Verification items for the finished model (mm, model axes). A direction names the side the tool comes from. Round coordinates to 2 decimals unless told otherwise and drop trailing zeros. Write each loop counter-clockwise with the first axis right and the second up, starting at its lowest first coordinate (ties: lowest second). Pieces come first, ordered by that corner, then holes. Notation, with made-up numbers: M 71.25,-5 L 97.25,-5 A27 ccw 97.25,19 Z; hole C 33.25,84.25 d1. An arc over 180 degrees is marked long. Answer in a Markdown table with one row per item. Add a question column.
1. Sectioned sample at A-A on y = 63.5. Record the cut outline in (x, z).
2. Go/stop test with flat-tipped pins: pin 1 Ø3.5 at (x, y) = (-41, 63.5) entering from -Z; pin 2 Ø1.6 at (y, z) = (67.5, -8) entering from -X; pin 3 Ø6 at (x, z) = (-35, -6) entering from -Y. Record where each tip stops, or that it passes through.
3. Sectioned sample at C-C on z = -7.25. Record the cut outline in (x, y).
4. Sectioned sample at D-D on x = -54. Record the cut outline in (y, z), plus the area to 3 significant figures.
5. Sectioned sample at B-B on x = -27. Record the cut outline in (y, z).
6. Draft check along Y on faces 1 (the cylindrical face through (-48.162, 64.215, 3.944)), 2 (the cylindrical face through (-23.918, 70.401, -2.14)), 3 (the flat face through (-27, 68, -12)), 4 (the flat face through (-27.37, 65.96, -11.51)). Enter one of: pulls with the +Y half, pulls with the -Y half, needs draft (parallel to the pull), parting line crosses it, or undercut.
7. Material ranges on probe 1 along Z at (x, y) = (-58, 63.5); probe 2 along X at (y, z) = (67, -5.75); probe 3 along Y at (x, z) = (-29, -3), recorded low to high.
8. Set-up check for faces 5 (the flat face through (-27.37, 69.96, -11.49)), 6 (the cylindrical face through (-30.746, 65.573, -6.084)), 7 (the flat face through (-33, 64.971, 3)), 8 (the cylindrical face through (-30.715, 70.401, -6.084)), 9 (the flat face through (-31.316, 68, -6)): record each of +Z, -Z, +X, -X, +Y, -Y from which the full face is reachable in a straight line by a thin tool's end or side.
```python
from build123d import *

# Parameters (mm, degrees)
BOSS_EXTRUDE1_DEPTH = 8
BOSS_EXTRUDE2_DEPTH = 12
SKETCH3_R           = 2
CUT_EXTRUDE1_DEPTH  = 8
FILLET1_R           = 2
CUT_EXTRUDE2_DEPTH  = 8


with BuildPart() as part:
    # Sketch1 → Boss-Extrude1 (new body)
    with BuildSketch(Plane.XY):
        with BuildLine():
            Line((-23.31623588, 68.971177363), (-23.31623588, 70.971177363))
            Line((-23.31623588, 70.971177363), (-55.31623588, 70.971177363))
            ThreePointArc((-55.31623588, 70.971177363), (-60.433053073, 61.837779556), (-49.971894623, 62.243904636))
            ThreePointArc((-49.971894623, 62.243904636), (-48.129441748, 64.23519169), (-45.518276909, 64.971177363))
            Line((-45.518276909, 64.971177363), (-23.31623588, 64.971177363))
            Line((-23.31623588, 64.971177363), (-23.31623588, 68.971177363))
        make_face()
    extrude(amount=BOSS_EXTRUDE1_DEPTH)

    # Sketch2 → Boss-Extrude2 (add)
    with BuildSketch(Plane.XY):
        Polygon((-23.31623588, 68.971177363), (-23.31623588, 70.971177363), (-31.31623588, 70.971177363), (-31.31623588, 67.971177363), (-31.31623588, 64.971177363), (-23.31623588, 64.971177363), align=None)
    extrude(amount=-BOSS_EXTRUDE2_DEPTH)

    # Sketch3 → Cut-Extrude1 (cut)
    with BuildSketch(Plane(origin=(0, 0, 0), x_dir=(-1, 0, 0), z_dir=(0, 0, -1))):
        with Locations((55.31623588, 64.971177363)):
            Circle(SKETCH3_R)
    extrude(amount=-CUT_EXTRUDE1_DEPTH, mode=Mode.SUBTRACT)

    # Fillet1
    fillet1_edges = [part.edges().sort_by_distance(p)[0] for p in [
        (-31.31623588, 70.971177363, -6),
        (-31.31623588, 64.971177363, -6),
        (-23.31623588, 64.971177363, -2),
        (-23.31623588, 70.971177363, -2),
    ]]
    fillet(fillet1_edges, radius=FILLET1_R)

    # Sketch4 → Cut-Extrude2 (cut)
    with BuildSketch(Plane.ZY.offset(31.31623588)):
        Polygon((-12, 70.971177363), (-13, 70.971177363), (-13, 64.971177363), (-12, 64.971177363), (-12, 65.471177363), (-11, 66.471177363), (-12, 67.471177363), (-12, 68.471177363), (-11, 69.471177363), (-12, 70.471177363), align=None)
    extrude(amount=-CUT_EXTRUDE2_DEPTH, mode=Mode.SUBTRACT)


solid = part.part
```
Geometry check:
| question | item | result |
|---|---|---|
| 1 | outline | M -61.13,0 L -56.67,0 L -56.67,8 L -61.13,8 Z; M -53.96,0 L -49.06,0 L -49.06,8 L -53.96,8 Z |
| 2 | pin 1 | stops at z = 0 |
| 2 | pin 2 | stops at x = -31.32 |
| 2 | pin 3 | passes through |
| 3 | outline | M -31.32,66.97 A2 ccw -29.32,64.97 L -25.32,64.97 A2 ccw -23.32,66.97 L -23.32,68.97 A2 ccw -25.32,70.97 L -29.32,70.97 A2 ccw -31.32,68.97 Z |
| 4 | outline | M 59.12,0 L 63.47,0 L 63.47,8 L 59.12,8 Z; M 66.48,0 L 70.97,0 L 70.97,8 L 66.48,8 Z |
| 4 | area | 70.7 mm2 |
| 5 | outline | M 64.97,-12 L 65.47,-12 L 66.47,-11 L 67.47,-12 L 68.47,-12 L 69.47,-11 L 70.47,-12 L 70.97,-12 L 70.97,8 L 64.97,8 Z |
| 6 | face 1 | pulls with the -Y half |
| 6 | face 2 | pulls with the +Y half |
| 6 | face 3 | needs draft |
| 6 | face 4 | undercut |
| 7 | probe 1 | z = 0 to 8 |
| 7 | probe 2 | x = -31.32 to -23.32 |
| 7 | probe 3 | y = 64.97 to 70.97 |
| 8 | face 5 | -Z, +X, -X |
| 8 | face 6 | -Z, -X, -Y |
| 8 | face 7 | +Z, -Z, +X, -Y |
| 8 | face 8 | -Z, -X, +Y |
| 8 | face 9 | -Z, -X, +Y, -Y |
